For this review, use the dimensioned drawing (mm, ordinates from the lowest corner) and the shaded views. A direction names the side the tool comes from. Coordinates: 2 decimals unless noted, no trailing zeros. Order: outer loops, then holes, each group sorted by start corner. A loop starts at its lowest first (then second) coordinate and runs counter-clockwise, first axis right, second up. Notation, with made-up numbers: M 10,12.5 L 47,12.5 A30 ccw 47,39.5 Z; hole C 11.5,-29.75 d7. An arc over 180 degrees is marked long. Answer as CSV lines item,"result". Start each with the question number.
Q1. Consider section C-C on z = 3.15. Write out the cut boundary in (x, y).
Q2. The part is to be moulded in two halves that separate along Y. For the marked faces 3, 4, 5 and 6, say which applies: +Y half, -Y half, draft (parallel to the pull), parting line (faces both ways), or undercut.
Q3. Machinability: for the marked faces 1 and 2, which of the approach directions +Z, -Z, +X, -X, +Y, -Y give a long, thin tool a straight path to every point of the face, cutting with its end or side? Answer none if there is none.
Q4. Wall thickness on L1, parallel to Y at x = 25, z = 3.25; L2, parallel to X at y = 14.75, z = 2.25; L3, parallel to Z at x = 16, y = 22.25: over which ranges is each line inside the solid? List them lowest first. Write a range as [from, to].
Q5. Consider section A-A on x = 21. Write out the cut boundary in (y, z), and give its area (3 significant figures).
Q6. For P1, Ø2, axis at x = 7.5, y = 8.5, coming from the +Z side; P2, Ø12, axis at x = 17, y = 5, coming from the +Z side, all flat-tipped, find the tip position at first contact; note any pin that passes through.
Q7. Consider section B-B on y = 18.5. Write out the cut boundary in (x, z), and give its area (3 significant figures).
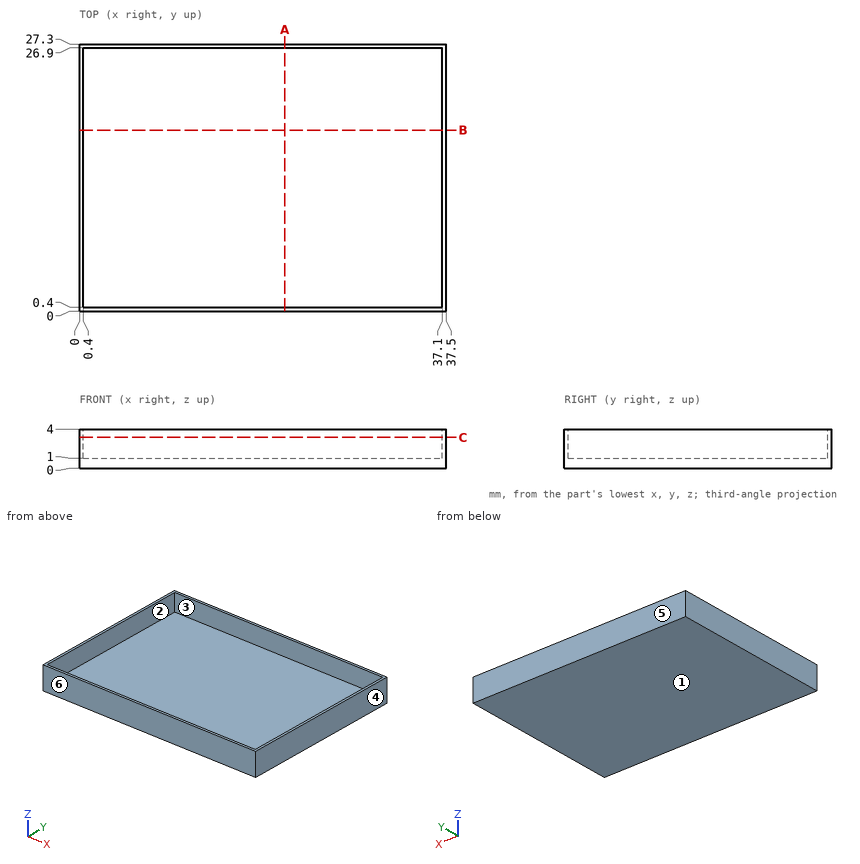
Evaluation:
1,outline,"M 0,0 L 37.5,0 L 37.5,27.3 L 0,27.3 Z; hole M 0.4,0.4 L 37.1,0.4 L 37.1,26.9 L 0.4,26.9 Z"
2,face 3,"undercut"
2,face 4,"draft"
2,face 5,"+Y half"
2,face 6,"-Y half"
3,face 1,"-Z, +X, -X, +Y, -Y"
3,face 2,"+Z"
4,L1,"y = [0, 0.4], [26.9, 27.3]"
4,L2,"x = [0, 0.4], [37.1, 37.5]"
4,L3,"z = [0, 1]"
5,outline,"M 0,0 L 27.3,0 L 27.3,4 L 26.9,4 L 26.9,1 L 0.4,1 L 0.4,4 L 0,4 Z"
5,area,"29.7 mm²"
6,P1,"stops at z = 1"
6,P2,"stops at z = 4"
7,outline,"M 0,0 L 37.5,0 L 37.5,4 L 37.1,4 L 37.1,1 L 0.4,1 L 0.4,4 L 0,4 Z"
7,area,"39.9 mm²"
